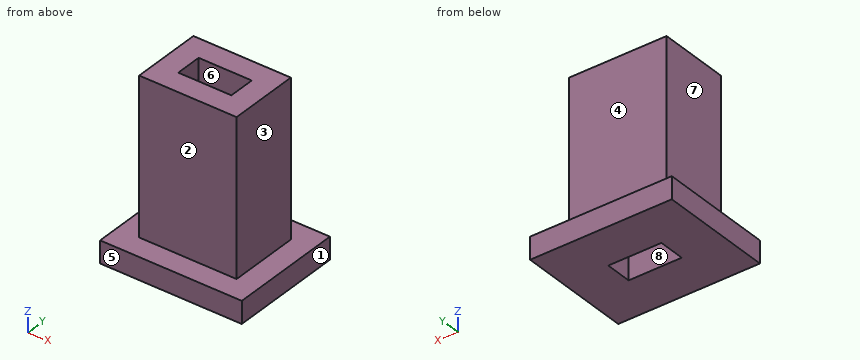
```python
from build123d import *

# Parameters (mm, degrees)
SKETCH_1_W      = 44
SKETCH_1_H      = 32
SKETCH_1_W_2    = 24
SKETCH_1_H_2    = 12
EXTRUDE_1_DEPTH = 80
SKETCH_2_W      = 64
SKETCH_2_H      = 52
SKETCH_2_W_2    = 44
SKETCH_2_H_2    = 32
EXTRUDE_2_DEPTH = 10


with BuildPart() as part:
    # 草图1 → 凸台-拉伸1 (new body)
    with BuildSketch(Plane.XY):
        Rectangle(SKETCH_1_W, SKETCH_1_H)
        Rectangle(SKETCH_1_W_2, SKETCH_1_H_2, mode=Mode.SUBTRACT)
    extrude(amount=EXTRUDE_1_DEPTH)

    # 草图2 → 凸台-拉伸2 (add)
    with BuildSketch(Plane(origin=(0, 0, 0), x_dir=(-1, 0, 0), z_dir=(0, 0, -1))):
        Rectangle(SKETCH_2_W, SKETCH_2_H)
        Rectangle(SKETCH_2_W_2, SKETCH_2_H_2, mode=Mode.SUBTRACT)
    extrude(amount=-EXTRUDE_2_DEPTH)


solid = part.part
```
Work out the finished part from the listing and answer in its coordinate system (mm). Face numbers are marked on the shaded views. A direction names the side the tool comes from. Give positions to 0.01 mm unless a question says otherwise; leave off trailing zeros. Write each loop counter-clockwise with the first axis right and the second up, starting at its lowest first coordinate (ties: lowest second). Pieces come first, ordered by that corner, then holes.
(1) The part is cut by section C-C on z = 59.5. Write down the section's boundary in (x, y).
Final values:
outline: (-22, -16) - (22, -16) - (22, 16) - (-22, 16) - close; hole (-12, -6) - (12, -6) - (12, 6) - (-12, 6) - close
(2) The part is cut by section D-D on y = -11.5. Write down the section's boundary in (x, z).
Final values:
outline: (-32, 0) - (32, 0) - (32, 10) - (22, 10) - (22, 80) - (-22, 80) - (-22, 10) - (-32, 10) - close
(3) The part is cut by section A-A on y = -3. Write down the section's boundary in (x, z).
Final values:
outline: (-32, 0) - (-12, 0) - (-12, 80) - (-22, 80) - (-22, 10) - (-32, 10) - close; (12, 0) - (32, 0) - (32, 10) - (22, 10) - (22, 80) - (12, 80) - close
(4) The part is cut by section B-B on x = -10. Write down the section's boundary in (y, z).
Final values:
outline: (-26, 0) - (-6, 0) - (-6, 80) - (-16, 80) - (-16, 10) - (-26, 10) - close; (6, 0) - (26, 0) - (26, 10) - (16, 10) - (16, 80) - (6, 80) - close
(5) The mould has two halves that part along X. Classify the marked faces 5, 6, 7 and 8: pulls with the +X half, pulls with the -X half, needs draft (parallel to the pull), parting line crosses it, or undercut.
Final values:
face 5: needs draft
face 6: undercut
face 7: pulls with the -X half
face 8: undercut
(6) Flat-ended cylindrical pins translate along their axes: pin 1 Ø1.5 at (x, y) = (-1, -17) entering from -Z; pin 2 Ø3 at (x, z) = (13, 32.5) entering from -Y; pin 3 Ø3 at (x, z) = (0.5, 48.5) entering from +Y; pin 4 Ø9.5 at (y, z) = (2, 43.5) entering from +X. Find the tip coordinate at first contact, or state that the pin passes through.
Final values:
pin 1: stops at z = 0
pin 2: stops at y = -16
pin 3: stops at y = 16
pin 4: stops at x = 22
(7) Straight lines are drawn through the part: line 1 (Y direction, x = 2, z = 49); line 2 (X direction, y = -5, z = 29); line 3 (X direction, y = -5, z = 9). For each, find the intervals that lie inside material, in ascending order.
Final values:
line 1: y = -16 to -6, 6 to 16
line 2: x = -22 to -12, 12 to 22
line 3: x = -32 to -12, 12 to 32
(8) Which of the six approach directions +Z, -Z, +X, -X, +Y, -Y give full straight-line access (tool end or side, diameter ignored) to the marked faces 1, 2, 3 and 4?
Final values:
face 1: +Z, -Z, +X, +Y, -Y
face 2: +Z, +X, -X, -Y
face 3: +Z, +X, +Y, -Y
face 4: +Z, +X, -X, +Y
